```python
from build123d import *

# Parameters (mm, degrees)
BOSS_EXTRUDE1_DEPTH  = 40
CUT_EXTRUDE1_REACH   = 80.602
SKETCH2_R            = 2.5
CUT_EXTRUDE2_DEPTH   = 10
SKETCH6_W            = 55
SKETCH6_H            = 110
BOSS_EXTRUDE8_DEPTH  = 8
CUT_EXTRUDE3_REACH   = 117.156
SKETCH7_W            = 4
SKETCH7_H            = 10
BOSS_EXTRUDE9_DEPTH  = 20
BOSS_EXTRUDE10_START = -48
BOSS_EXTRUDE10_DEPTH = 7
RIB1_REACH           = 120.495
SKETCH10_WALL_W      = 267.27372249
SKETCH10_WALL_H      = 8


with BuildPart() as part:
    # Sketch1 → Boss-Extrude1 (new body)
    with BuildSketch(Plane.XY):
        Polygon((-21, 0), (21, 0), (21, 42), (1.5, 42), (1.5, 58.5), (6.5, 58.5), (6.5, 48.5), (27.5, 48.5), (27.5, -6.5), (-27.5, -6.5), (-27.5, 48.5), (-6.5, 48.5), (-6.5, 58.5), (-1.5, 58.5), (-1.5, 42), (-21, 42), align=None)
    extrude(amount=BOSS_EXTRUDE1_DEPTH)

    # Cut-Extrude1: up to this face of the body (flat: up to its plane)
    cut_extrude1_end = Plane(part.part.faces().sort_by_distance((6.5, 53.5, 20))[0])
    # Sketch2 → Cut-Extrude1 (cut, up to the picked face)
    with BuildSketch(Plane.ZY.offset(6.5), mode=Mode.PRIVATE) as cut_extrude1_sk1:
        with Locations(Location((11, 53.5, 0), (0, 0, 270))):
            Circle(SKETCH2_R)
    cut_extrude1_tool1 = split(extrude(cut_extrude1_sk1.sketch, amount=-CUT_EXTRUDE1_REACH, mode=Mode.PRIVATE), bisect_by=cut_extrude1_end, keep=Keep.BOTH, mode=Mode.PRIVATE)
    # Sketch2 → Cut-Extrude1 (cut, up to the picked face)
    with BuildSketch(Plane.ZY.offset(6.5), mode=Mode.PRIVATE) as cut_extrude1_sk2:
        with Locations(Location((29, 53.5, 0), (0, 0, 270))):
            Circle(SKETCH2_R)
    cut_extrude1_tool2 = split(extrude(cut_extrude1_sk2.sketch, amount=-CUT_EXTRUDE1_REACH, mode=Mode.PRIVATE), bisect_by=cut_extrude1_end, keep=Keep.BOTH, mode=Mode.PRIVATE)
    add(cut_extrude1_tool1.solids().sort_by(Axis((-6.5, 53.5, 11), (1, 0, 0)))[0], mode=Mode.SUBTRACT)
    add(cut_extrude1_tool2.solids().sort_by(Axis((-6.5, 53.5, 29), (1, 0, 0)))[0], mode=Mode.SUBTRACT)

    # Sketch3 → Cut-Extrude2 (cut)
    with BuildSketch(Plane(origin=(0, 0, 0), x_dir=(-1, 0, 0), z_dir=(0, 0, -1))):
        with BuildLine():
            Line((20.5, -6.5), (19.170549473, -5.005824209))
            ThreePointArc((19.170549473, -5.005824209), (18.157592064, -4.262982703), (16.929285786, -4))
            Line((16.929285786, -4), (-3.929285786, -4))
            ThreePointArc((-3.929285786, -4), (-5.157592064, -4.262982703), (-6.170549473, -5.005824209))
            Line((-6.170549473, -5.005824209), (-7.5, -6.5))
            Line((-7.5, -6.5), (20.5, -6.5))
        make_face()
    extrude(amount=-CUT_EXTRUDE2_DEPTH, mode=Mode.SUBTRACT)

    # Cut-Extrude3: up to this face of the body (flat: up to its plane)
    cut_extrude3_end = Plane(part.part.faces().sort_by_distance((6.5, 53.5, 20))[0])
    # Sketch7 → Cut-Extrude3 (cut, up to the picked face)
    with BuildSketch(Plane.ZY.offset(6.5), mode=Mode.PRIVATE) as cut_extrude3_sk1:
        with Locations((38, 53.5)):
            Rectangle(SKETCH7_W, SKETCH7_H)
    cut_extrude3_tool1 = split(extrude(cut_extrude3_sk1.sketch, amount=-CUT_EXTRUDE3_REACH, mode=Mode.PRIVATE), bisect_by=cut_extrude3_end, keep=Keep.BOTH, mode=Mode.PRIVATE)
    # Sketch7 → Cut-Extrude3 (cut, up to the picked face)
    with BuildSketch(Plane.ZY.offset(6.5), mode=Mode.PRIVATE) as cut_extrude3_sk2:
        with Locations((2, 53.5)):
            Rectangle(SKETCH7_W, SKETCH7_H)
    cut_extrude3_tool2 = split(extrude(cut_extrude3_sk2.sketch, amount=-CUT_EXTRUDE3_REACH, mode=Mode.PRIVATE), bisect_by=cut_extrude3_end, keep=Keep.BOTH, mode=Mode.PRIVATE)
    add(cut_extrude3_tool1.solids().sort_by(Axis((-6.5, 53.5, 38), (1, 0, 0)))[0], mode=Mode.SUBTRACT)
    add(cut_extrude3_tool2.solids().sort_by(Axis((-6.5, 53.5, 2), (1, 0, 0)))[0], mode=Mode.SUBTRACT)



with BuildPart() as body_2:
    # Sketch6 → Boss-Extrude8 (new body)
    with BuildSketch(Plane.XY.offset(40)):
        with Locations((0, 44)):
            Rectangle(SKETCH6_W, SKETCH6_H)
    extrude(amount=BOSS_EXTRUDE8_DEPTH)


with BuildPart() as part_1:
    add(part.part)

    add(body_2.part)  # Boss-Extrude9 merges body 2
    # Sketch9 → Boss-Extrude9 (add)
    with BuildSketch(Plane(origin=(27.5, 0, 0), x_dir=(0, 0, -1), z_dir=(1, 0, 0))):
        Polygon((-40, -14.5), (-48, -11), (-40, -11), (-40, -6.5), (-10, -6.5), (-10, -14.5), align=None)
    extrude(amount=-BOSS_EXTRUDE9_DEPTH)

    # Sketch9<2> → Boss-Extrude10 (add)
    with BuildSketch(Plane(origin=(27.5, 0, 0), x_dir=(0, 0, -1), z_dir=(1, 0, 0)).offset(BOSS_EXTRUDE10_START)):
        Polygon((-40, -14.5), (-48, -11), (-40, -11), (-40, -6.5), (-10, -6.5), (-10, -14.5), align=None)
    extrude(amount=-BOSS_EXTRUDE10_DEPTH)

    # Sketch10 wall → Rib1 (add, up to next)
    with BuildSketch(Plane(origin=(16.5, 58.5, 30), x_dir=(0, -0.707106781187, -0.707106781187), z_dir=(0, 0.707106781187, -0.707106781187)), mode=Mode.PRIVATE) as rib1_sk1:
        Rectangle(SKETCH10_WALL_W, SKETCH10_WALL_H)
    rib1_tool1 = extrude(rib1_sk1.sketch, amount=-RIB1_REACH, mode=Mode.PRIVATE) - part_1.part
    rib1 = rib1_tool1.solids().sort_by_distance((16.5, 58.5, 30))[0]
    add(rib1)

    # Mirror1: Rib1 across plane
    add(rib1.mirror(Plane(origin=(0, 0, 0), x_dir=(0, 0, 1), z_dir=(1, 0, 0))))


solid = part_1.part
```
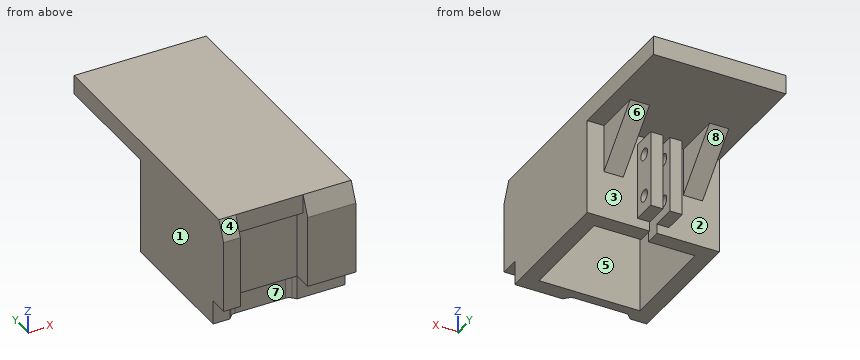
Here's how the part is built. I have some questions about the finished solid (model axes, mm). Face numbers are marked on the shaded views. A direction names the side the tool comes from. Coordinates: 2 decimals unless noted, no trailing zeros. Loops run counter-clockwise (first coordinate to the right, second up) from the corner with the lowest first, then second, coordinate; pieces in that order, holes last. Notation, with made-up numbers: M 43.25,10 L 92.25,10 A10 ccw 92.25,16 Z; hole C 49.25,-12.75 d2. An arc over 180 degrees is marked long. One line per item, written item: value.
1. Imagine slicing it at A-A (y = 66). List the corners of the cut face in (x, z) for me, and give its area (3 significant figures).
Geometry says:
outline: M -27.5,40 L -20.5,40 L -20.5,37.5 L -12.5,37.5 L -12.5,40 L 12.5,40 L 12.5,37.5 L 20.5,37.5 L 20.5,40 L 27.5,40 L 27.5,48 L -27.5,48 Z
area: 480 mm2
2. Imagine slicing it at D-D (z = 29). State how many separate pieces and enclosed holes the cut face has, and give its area (3 significant figures).
Geometry says:
separate pieces: 3
enclosed holes: 0
area: 1,650 mm2
3. On a 3-axis mill with a long thin cutter (end or side, diameter ignored), from which of +Z, -Z, +X, -X, +Y, -Y can I reach the whole of each face in a straight line? I mean the marked faces 5, 6, 7 and 8. Say none if no direction works.
Geometry says:
face 5: -Z
face 6: -Z, +X, +Y
face 7: -Z, -Y
face 8: -Z, -X, +Y
4. Will these pins go through, and if not, where does the flat tip stop? pin 1 Ø2 at (x, y) = (4, 83.5) entering from -Z; pin 2 Ø1.5 at (x, z) = (4.5, 19) entering from +Y; pin 3 Ø2 at (x, z) = (11, 5.5) entering from +Y.
Geometry says:
pin 1: stops at z = 40
pin 2: stops at y = 58.5
pin 3: stops at y = 48.5
5. Please list where these lines run through material, in increasing order: probe 1 along Z at (x, y) = (4.25, 53.5); probe 2 along Y at (x, z) = (10, 5); probe 3 along X at (y, z) = (-9, 32).
Geometry says:
probe 1: z = 4 to 8.5, 13.5 to 26.5, 31.5 to 36, 40 to 48
probe 2: y = -6.5 to 0, 42 to 48.5
probe 3: x = -27.5 to -20.5, 7.5 to 27.5
6. Thinking about a two-plate mould opening in X: for the marked faces 1, 2, 3 and 4, which applies, +X half, -X half, draft (parallel to the pull), parting line (faces both ways), or undercut?
Geometry says:
face 1: -X half
face 2: undercut
face 3: undercut
face 4: draft
7. Imagine slicing it at B-B (z = 24). List the corners of the cut face in (x, y) for me.
Geometry says:
outline: M -27.5,-14.5 L -20.5,-14.5 L -20.5,-6.5 L 7.5,-6.5 L 7.5,-14.5 L 27.5,-14.5 L 27.5,48.5 L 20.5,48.5 L 20.5,52.5 L 12.5,52.5 L 12.5,48.5 L 6.5,48.5 L 6.5,58.5 L 1.5,58.5 L 1.5,42 L 21,42 L 21,0 L -21,0 L -21,42 L -1.5,42 L -1.5,58.5 L -6.5,58.5 L -6.5,48.5 L -12.5,48.5 L -12.5,52.5 L -20.5,52.5 L -20.5,48.5 L -27.5,48.5 Z
8. Imagine slicing it at C-C (x = 11). List the corners of the cut face in (y, z) for me.
Geometry says:
outline: M -14.5,10 L -6.5,10 L -6.5,0 L 0,0 L 0,40 L 42,40 L 42,0 L 48.5,0 L 48.5,40 L 99,40 L 99,48 L -11,48 L -14.5,40 Z
